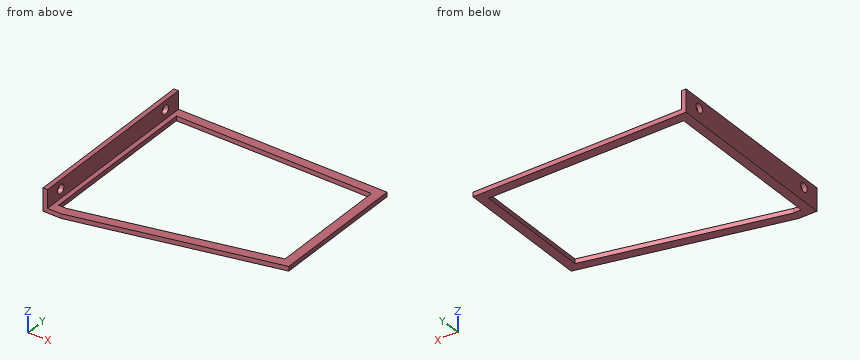
from build123d import *

# Parameters (mm, degrees)
BOSS_EXTRUDE1_DEPTH = 5
SKETCH2_W           = 5
SKETCH2_H           = 200
BOSS_EXTRUDE2_DEPTH = 20
SKETCH3_R           = 5
CUT_EXTRUDE1_DEPTH  = 307.481412279


with BuildPart() as part:
    # Sketch1 → Boss-Extrude1 (new body)
    with BuildSketch(Plane.XY):
        Polygon((0, 0), (20, 0), (235.880609996, 50), (235.880609996, 200), (0, 200), align=None)
        Polygon((10, 190), (225.880609996, 190), (225.880609996, 57.948616206), (18.857079694, 10), (10, 10), align=None, mode=Mode.SUBTRACT)
    extrude(amount=BOSS_EXTRUDE1_DEPTH)

    # Sketch2 → Boss-Extrude2 (add)
    with BuildSketch(Plane.XY.offset(5)):
        with Locations((2.5, 100)):
            Rectangle(SKETCH2_W, SKETCH2_H)
    extrude(amount=BOSS_EXTRUDE2_DEPTH)

    # Sketch3 → Cut-Extrude1 (cut, through all)
    with BuildSketch(Plane(origin=(5, 0, 0), x_dir=(0, 0, -1), z_dir=(1, 0, 0))):
        with Locations(Location((-15, 180, 0), (0, 0, 90))):
            Circle(SKETCH3_R)
        with Locations(Location((-15, 20, 0), (0, 0, 90))):
            Circle(SKETCH3_R)
    extrude(amount=-CUT_EXTRUDE1_DEPTH, mode=Mode.SUBTRACT)


solid = part.part
Geometry: final body of the model. Coordinates: model frame, mm. Coordinates: 2 decimals unless noted, no trailing zeros. Loops run counter-clockwise (first coordinate to the right, second up) from the corner with the lowest first, then second, coordinate; pieces in that order, holes last. Notation, with made-up numbers: (77.5, -3) - (127.5, -3) arc R34 ccw to (127.5, 30) - close; hole circle Ø7 at (30, 86.25). An arc over 180 degrees is marked (long way). Put each result on its own line as item: value. Start each with the question number.
Q1. Line query: line 1 (Z direction, x = 2, y = 180); line 2 (Z direction, x = 181, y = 39). Output: solid intervals per line, ascending.
Q2. Cut plane B-B, the plane z = 15. Return loops of the section in (x, y).
Q3. Cut plane A-A, the plane y = 94. Return loops of the section in (x, z).
Q4. Pin query (flat end, axial travel): pin 1 Ø4 at (y, z) = (105.5, 2) entering from -X; pin 2 Ø2.5 at (x, z) = (103.5, 2.5) entering from -Y; pin 3 Ø11.5 at (y, z) = (180, 15) entering from +X. Return the tip coordinate at first contact, or that it passes through.
Q5. Cut plane C-C, the plane x = 190.5. Return loops of the section in (y, z).
Q6. Cut plane D-D, the plane y = 180. Return loops of the section in (x, z).
Filled sheet:
1. line 1: 0 to 10, 20 to 25
1. line 2: 0 to 5
2. outline: (0, 0) - (5, 0) - (5, 15) - (0, 15) - close; (0, 25) - (5, 25) - (5, 175) - (0, 175) - close; (0, 185) - (5, 185) - (5, 200) - (0, 200) - close
3. outline: (0, 0) - (10, 0) - (10, 5) - (5, 5) - (5, 25) - (0, 25) - close; (225.88, 0) - (235.88, 0) - (235.88, 5) - (225.88, 5) - close
4. pin 1: x = 0
4. pin 2: y = 19.05
4. pin 3: x = 5
5. outline: (39.49, 0) - (49.75, 0) - (49.75, 5) - (39.49, 5) - close; (190, 0) - (200, 0) - (200, 5) - (190, 5) - close
6. outline: (0, 0) - (10, 0) - (10, 5) - (5, 5) - (5, 10) - (0, 10) - close; (0, 20) - (5, 20) - (5, 25) - (0, 25) - close; (225.88, 0) - (235.88, 0) - (235.88, 5) - (225.88, 5) - close
